from build123d import *

# Parameters (mm, degrees)
BASE_W                                       = 90
BASE_H                                       = 62.5
BASE_EXTRUDE_DEPTH                           = 2
WALLS_W                                      = 90
WALLS_H                                      = 62.5
WALLS_W_2                                    = 86
WALLS_H_2                                    = 58.5
WALLS_EXTRUDE_DEPTH                          = 64
OUTJUT_EXTRUDE_DEPTH                         = 8
HOLES_R                                      = 1.15
HOLES_CUT_DEPTH                              = 6
ANTENNA_GPS_HOLES_R                          = 3.25
ANTENNA_GPS_HOLES_CUT_DEPTH                  = 2
PAD_W                                        = 106
PAD_H                                        = 78.5
PAD_EXTRUDE_DEPTH                            = 4
SCREW_HOLES_R                                = 1.5
SCREW_HOLES_CUT_DEPTH                        = 5
WALL_FILLETS_R                               = 1.5
LENGTH_SUPPORTS_EXTRUDE_DEPTH                = 1
LENGTH_SUPPORT_EXTRUDE_OPPOSING_MIRR_2_DEPTH = 1
WIDTH_SUPPORTS_EXTRUDE_DEPTH                 = 1
WIDTH_SUPPORTS_EXTRUDE_OPPOSING_MIRR_2_DEPTH = 1
ZIP_TIE_HOLE_W                               = 4.5
ZIP_TIE_HOLE_H                               = 4.5
ZIP_TIE_HOLE_LENGTH_CUT_DEPTH                = 5
ZIP_TIE_HOLE_LENGTH_OPPOSING_MIRROR_COPY_W   = 4.5
ZIP_TIE_HOLE_LENGTH_OPPOSING_MIRROR_COPY_H   = 4.5
ZIP_TIE_HOLE_LENGTH_OPPOSING_MIRROR_2_DEPTH  = 5
ZIP_TIE_HOLE_WIDTH_W                         = 4.5
ZIP_TIE_HOLE_WIDTH_H                         = 4.5
ZIP_TIE_HOLE_WIDTH_CUT_DEPTH                 = 5
ZIP_TIE_HOLE_WIDTH_OPPOSING_MIRROR_COPY_W    = 4.5
ZIP_TIE_HOLE_WIDTH_OPPOSING_MIRROR_COPY_H    = 4.5
ZIP_TIE_HOLE_WIDTH_OPPOSING_MIRROR_C_2_DEPTH = 5
ZIP_TIE_FILLETS_R                            = 2.5
PAD_FILLETS_R                                = 2.5


with BuildPart() as part:
    # Base → Base Extrude (new body)
    with BuildSketch(Plane(origin=(0, 0, 0), x_dir=(1, 0, 0), z_dir=(0, 1, 0))):
        with Locations((45, 31.25)):
            Rectangle(BASE_W, BASE_H)
    extrude(amount=BASE_EXTRUDE_DEPTH)

    # Walls → Walls Extrude (add)
    with BuildSketch(Plane(origin=(0, 2, 0), x_dir=(1, 0, 0), z_dir=(0, 1, 0))):
        with Locations((45, 31.25)):
            Rectangle(WALLS_W, WALLS_H)
        with Locations((45, 31.25)):
            Rectangle(WALLS_W_2, WALLS_H_2, mode=Mode.SUBTRACT)
    extrude(amount=WALLS_EXTRUDE_DEPTH)

    # Outjut → Outjut Extrude (add)
    with BuildSketch(Plane(origin=(0, 66, 0), x_dir=(1, 0, 0), z_dir=(0, 1, 0))):
        with BuildLine():
            Line((0, 62.5), (6, 62.5))
            ThreePointArc((6, 62.5), (3, 65.5), (0, 62.5))
        make_face()
        with BuildLine():
            Line((90, 62.5), (84, 62.5))
            ThreePointArc((84, 62.5), (87, 65.5), (90, 62.5))
        make_face()
        with BuildLine():
            Line((90, 0), (84, 0))
            ThreePointArc((84, 0), (87, -3), (90, 0))
        make_face()
        with BuildLine():
            Line((0, 0), (6, 0))
            ThreePointArc((6, 0), (3, -3), (0, 0))
        make_face()
    extrude(amount=-OUTJUT_EXTRUDE_DEPTH)

    # Holes → Holes Cut (cut)
    with BuildSketch(Plane(origin=(0, 66, 0), x_dir=(1, 0, 0), z_dir=(0, 1, 0))):
        with Locations((3, 62.5)):
            Circle(HOLES_R)
        with Locations((87, 62.5)):
            Circle(HOLES_R)
        with Locations((87, 0)):
            Circle(HOLES_R)
        with Locations((3, 0)):
            Circle(HOLES_R)
    extrude(amount=-HOLES_CUT_DEPTH, mode=Mode.SUBTRACT)

    # Antenna/GPS Holes → Antenna/GPS Holes Cut (cut)
    with BuildSketch(Plane(origin=(0, 0, -62.5), x_dir=(-1, 0, 0), z_dir=(0, 0, -1))):
        with Locations((-23, 56.95)):
            Circle(ANTENNA_GPS_HOLES_R)
        with Locations((-67, 56.95)):
            Circle(ANTENNA_GPS_HOLES_R)
    extrude(amount=-ANTENNA_GPS_HOLES_CUT_DEPTH, mode=Mode.SUBTRACT)

    # Pad → Pad Extrude (add)
    with BuildSketch(Plane.XZ):
        with Locations((45, -31.25)):
            Rectangle(PAD_W, PAD_H)
    extrude(amount=-PAD_EXTRUDE_DEPTH)

    # Screw Holes → Screw Holes Cut (cut, through all)
    with BuildSketch(Plane(origin=(0, 4, 0), x_dir=(1, 0, 0), z_dir=(0, 1, 0))):
        with Locations((94, 66.5)):
            Circle(SCREW_HOLES_R)
        with Locations((-4, 66.5)):
            Circle(SCREW_HOLES_R)
        with Locations((94, -4)):
            Circle(SCREW_HOLES_R)
        with Locations((-4, -4)):
            Circle(SCREW_HOLES_R)
    extrude(amount=-SCREW_HOLES_CUT_DEPTH, mode=Mode.SUBTRACT)

    # Wall Fillets
    wall_fillets_edges = [part.edges().sort_by_distance(p)[0] for p in [
        (0, 31, 0),
        (0, 31, -62.5),
        (90, 31, -62.5),
        (90, 31, 0),
    ]]
    fillet(wall_fillets_edges, radius=WALL_FILLETS_R)

    # Length Supports → Length Supports Extrude (add, symmetric)
    with BuildSketch(Plane(origin=(22.5, 0, 0), x_dir=(0, 0, -1), z_dir=(1, 0, 0))):
        Polygon((0, 4), (-8, 4), (0, 10), align=None)
    length_supports_extrude = extrude(amount=LENGTH_SUPPORTS_EXTRUDE_DEPTH, both=True)

    # Length Support Extrude Mirror: Length Supports Extrude across plane
    add(length_supports_extrude.mirror(Plane(origin=(45, 0, 0), x_dir=(0, 0, 1), z_dir=(1, 0, 0))))

    # Length Support Extrude Opposing Mirror: Length Supports Extrude across plane
    add(length_supports_extrude.mirror(Plane.XY.offset(-31.25)))

    # Length Support Extrude Opposing Mirror c → Length Support Extrude Opposing Mirr 2 (add, symmetric)
    with BuildSketch(Plane(origin=(67.5, 0, -62.5), x_dir=(0, 0, 1), z_dir=(-1, 0, 0))):
        Polygon((0, 4), (-8, 4), (0, 10), align=None)
    extrude(amount=LENGTH_SUPPORT_EXTRUDE_OPPOSING_MIRR_2_DEPTH, both=True)

    # Width Supports → Width Supports Extrude (add, symmetric)
    with BuildSketch(Plane.XY.offset(-15.625)):
        Polygon((0, 4), (-8, 4), (0, 10), align=None)
    width_supports_extrude = extrude(amount=WIDTH_SUPPORTS_EXTRUDE_DEPTH, both=True)

    # Width Supports Extrude Mirror: Width Supports Extrude across plane
    add(width_supports_extrude.mirror(Plane.XY.offset(-31.25)))

    # Width Supports Extrude Opposing Mirror: Width Supports Extrude across plane
    add(width_supports_extrude.mirror(Plane(origin=(45, 0, 0), x_dir=(0, 0, 1), z_dir=(1, 0, 0))))

    # Width Supports Extrude Opposing Mirror c → Width Supports Extrude Opposing Mirr 2 (add, symmetric)
    with BuildSketch(Plane(origin=(90, 0, -46.875), x_dir=(-1, 0, 0), z_dir=(0, 0, -1))):
        Polygon((0, 4), (-8, 4), (0, 10), align=None)
    extrude(amount=WIDTH_SUPPORTS_EXTRUDE_OPPOSING_MIRR_2_DEPTH, both=True)

    # Zip Tie Hole → Zip Tie Hole Length Cut (cut, through all)
    with BuildSketch(Plane(origin=(0, 4, 0), x_dir=(1, 0, 0), z_dir=(0, 1, 0))):
        with Locations((39.75, -4)):
            Rectangle(ZIP_TIE_HOLE_W, ZIP_TIE_HOLE_H)
    zip_tie_hole_length_cut = extrude(amount=-ZIP_TIE_HOLE_LENGTH_CUT_DEPTH, mode=Mode.SUBTRACT)

    # Zip Tie Hole Length Mirror: Zip Tie Hole Length Cut across plane
    add(zip_tie_hole_length_cut.mirror(Plane(origin=(45, 0, 0), x_dir=(0, 0, 1), z_dir=(1, 0, 0))), mode=Mode.SUBTRACT)

    # Zip Tie Hole Length Opposing Mirror: Zip Tie Hole Length Cut across plane
    add(zip_tie_hole_length_cut.mirror(Plane.XY.offset(-31.25)), mode=Mode.SUBTRACT)

    # Zip Tie Hole Length Opposing Mirror copy → Zip Tie Hole Length Opposing Mirror  2 (cut, through all)
    with BuildSketch(Plane(origin=(90, 4, -62.5), x_dir=(-1, 0, 0), z_dir=(0, 1, 0))):
        with Locations((39.75, -4)):
            Rectangle(ZIP_TIE_HOLE_LENGTH_OPPOSING_MIRROR_COPY_W, ZIP_TIE_HOLE_LENGTH_OPPOSING_MIRROR_COPY_H)
    extrude(amount=-ZIP_TIE_HOLE_LENGTH_OPPOSING_MIRROR_2_DEPTH, mode=Mode.SUBTRACT)

    # Zip Tie Hole Width → Zip Tie Hole Width Cut (cut, through all)
    with BuildSketch(Plane(origin=(0, 4, 0), x_dir=(1, 0, 0), z_dir=(0, 1, 0))):
        with Locations((-4, 36.5)):
            Rectangle(ZIP_TIE_HOLE_WIDTH_W, ZIP_TIE_HOLE_WIDTH_H)
    zip_tie_hole_width_cut = extrude(amount=-ZIP_TIE_HOLE_WIDTH_CUT_DEPTH, mode=Mode.SUBTRACT)

    # Zip Tie Hole Width Mirror: Zip Tie Hole Width Cut across plane
    add(zip_tie_hole_width_cut.mirror(Plane.XY.offset(-31.25)), mode=Mode.SUBTRACT)

    # Zip Tie Hole Width Opposing Mirror: Zip Tie Hole Width Cut across plane
    add(zip_tie_hole_width_cut.mirror(Plane(origin=(45, 0, 0), x_dir=(0, 0, 1), z_dir=(1, 0, 0))), mode=Mode.SUBTRACT)

    # Zip Tie Hole Width Opposing Mirror copy → Zip Tie Hole Width Opposing Mirror c 2 (cut, through all)
    with BuildSketch(Plane(origin=(90, 4, -62.5), x_dir=(-1, 0, 0), z_dir=(0, 1, 0))):
        with Locations((-4, 36.5)):
            Rectangle(ZIP_TIE_HOLE_WIDTH_OPPOSING_MIRROR_COPY_W, ZIP_TIE_HOLE_WIDTH_OPPOSING_MIRROR_COPY_H)
    extrude(amount=-ZIP_TIE_HOLE_WIDTH_OPPOSING_MIRROR_C_2_DEPTH, mode=Mode.SUBTRACT)

    # Zip Tie Fillets
    zip_tie_fillets_edges = [part.edges().sort_by_distance(p)[0] for p in [
        (42, 4, 4),
        (48, 4, 4),
        (42, 4, -66.5),
        (48, 4, -66.5),
        (-4, 4, -34.25),
        (-4, 4, -28.25),
        (94, 4, -34.25),
        (94, 4, -28.25),
    ]]
    fillet(zip_tie_fillets_edges, radius=ZIP_TIE_FILLETS_R)

    # Pad Fillets
    pad_fillets_edges = [part.edges().sort_by_distance(p)[0] for p in [
        (-8, 2, -70.5),
        (-8, 2, 8),
        (98, 2, 8),
        (98, 2, -70.5),
    ]]
    fillet(pad_fillets_edges, radius=PAD_FILLETS_R)


solid = part.part
Design review of the part built by this model. Coordinates are the model's own, in mm. A direction names the side the tool comes from. Round coordinates to 2 decimals unless told otherwise and drop trailing zeros. Write each loop counter-clockwise with the first axis right and the second up, starting at its lowest first coordinate (ties: lowest second). Pieces come first, ordered by that corner, then holes.
Item 1: Draft analysis for pull direction X (two halves, no side actions). For faces 1 (the cylindrical face through (47.248, 3.287, 3.968)), 2 (the cylindrical face through (97, 2, -70)), 3 (the flat face through (44, 0, -31)), state which applies: released by +X, released by -X, zero draft, split by the parting line, or undercut.
Item 2: For faces 4 (the flat face through (23.5, 6, -65)), 5 (the flat face through (-2, 6, -16.625)), 6 (the flat face through (52.5, 2, -67)), list the 3-axis set-ups (+Z, -Z, +X, -X, +Y, -Y) from which the entire face can be reached by the end or side of a thin tool; tool diameter is ignored.
Item 3: Wall thickness on L1, parallel to Z at x = -4, y = 1.2; L2, parallel to Z at x = 87, y = 63; L3, parallel to X at y = 1.55, z = 4: over which ranges is each line inside the solid? List them lowest first.
Item 4: For pin 1 Ø3 at (y, z) = (7.5, -66) entering from -X; pin 2 Ø2 at (x, y) = (58, 16) entering from -Z; pin 3 Ø2 at (x, y) = (76.5, 25.5) entering from +Z, all flat-tipped, find the tip position at first contact; note any pin that passes through.
Item 5: Consider section D-D on x = 58. Give the boundary of the cut face in (y, z), and give its area (3 significant figures).
Item 6: Consider section B-B on y = 35.5. Give the boundary of the cut face in (x, z).
Item 7: Consider section C-C on z = -19. Give the boundary of the cut face in (x, y).
Item 8: Consider section A-A on x = 94. Count the separate pieces of the cut face and the enclosed holes in it, and give its area (3 significant figures).
Check values:
1. face 1: undercut
1. face 2: released by +X
1. face 3: zero draft
2. face 4: -Z, +Y
2. face 5: -X, +Y
2. face 6: +Y, -Y
3. L1: z = -70.5 to -68, -65 to -38.75, -34.25 to -28.25, -23.75 to 2.5, 5.5 to 8
3. L2: z = -65.5 to -63.65, -61.35 to -60.5, -2 to -1.15, 1.15 to 3
3. L3: x = -8 to -5.5, -2.5 to 37.5, 42 to 48, 52.5 to 92.5, 95.5 to 98
4. pin 1: stops at x = 21.5
4. pin 2: stops at z = -62.5
4. pin 3: stops at z = 0
5. outline: (0, -70.5) - (4, -70.5) - (4, -62.5) - (66, -62.5) - (66, -60.5) - (4, -60.5) - (4, -2) - (66, -2) - (66, 0) - (4, 0) - (4, 8) - (0, 8) - close
5. area: 562 mm2
6. outline: (0, -61) arc R1.5 ccw to (1.5, -62.5) - (88.5, -62.5) arc R1.5 ccw to (90, -61) - (90, -1.5) arc R1.5 ccw to (88.5, 0) - (1.5, 0) arc R1.5 ccw to (0, -1.5) - close; hole (2, -60.5) - (88, -60.5) - (88, -2) - (2, -2) - close
7. outline: (-8, 0) - (98, 0) - (98, 4) - (90, 4) - (90, 66) - (88, 66) - (88, 4) - (2, 4) - (2, 66) - (0, 66) - (0, 4) - (-8, 4) - close
8. separate pieces: 5
8. enclosed holes: 0
8. area: 263 mm2
